```python
from build123d import *

# Parameters (mm, degrees)
SKETCH1_R           = 0.95
BOSS_EXTRUDE1_DEPTH = 3
SKETCH2_R           = 4
SKETCH2_R_2         = 0.95
BOSS_EXTRUDE2_DEPTH = 58


with BuildPart() as part:
    # Sketch1 → Boss-Extrude1 (new body)
    with BuildSketch(Plane(origin=(0, 0, 0), x_dir=(1, 0, 0), z_dir=(0, 1, 0))):
        with BuildLine():
            Line((-4.153311931, -5), (4.153311931, -5))
            ThreePointArc((4.153311931, -5), (6.5, 0), (4.153311931, 5))
            Line((4.153311931, 5), (-4.153311931, 5))
            ThreePointArc((-4.153311931, 5), (-6.5, 0), (-4.153311931, -5))
        make_face()
        with Locations(Location((0, 0, 0), (0, 0, 270))):
            Circle(SKETCH1_R, mode=Mode.SUBTRACT)
    extrude(amount=BOSS_EXTRUDE1_DEPTH)

    # Sketch2 → Boss-Extrude2 (add)
    with BuildSketch(Plane(origin=(0, 3, 0), x_dir=(1, 0, 0), z_dir=(0, 1, 0))):
        with Locations(Location((0, 0, 0), (0, 0, 90))):
            Circle(SKETCH2_R)
        with Locations(Location((0, 0, 0), (0, 0, 270))):
            Circle(SKETCH2_R_2, mode=Mode.SUBTRACT)
    extrude(amount=BOSS_EXTRUDE2_DEPTH)


solid = part.part
```
Check sheet for the modelled part. Datum: model origin and axes. Units: mm. A direction names the side the tool comes from. Coordinates: 2 decimals unless noted, no trailing zeros. Order: outer loops, then holes, each group sorted by start corner. A loop starts at its lowest first (then second) coordinate and runs counter-clockwise, first axis right, second up. Notation, with made-up numbers: M -35,60.25 L -12,60.25 A20 cw -12,96.25 Z; hole C 0.5,1.5 d2. An arc over 180 degrees is marked long. One line per question, with ' | ' between items. Start each with the question number.
Item 1: Sectioned sample at A-A on z = 0. Record the cut outline in (x, y).
Item 2: Sectioned sample at D-D on z = -3.25. Record the cut outline in (x, y), and give its area (3 significant figures).
Item 3: Gauge pin test, flat ends, axial feed: P1, Ø2, axis at x = -2, y = 15, coming from the +Z side; P2, Ø1.5, axis at y = 21.5, z = 0, coming from the -X side; P3, Ø1.5, axis at y = 14, z = -2, coming from the +X side. Record the tip position at first contact, or that the pin passes through.
Item 4: Mould release check, pull along Z, two halves, no side actions. Record for faces 3 (the cylindrical face through (-0.36, 30.07, 0.88)), 4 (the flat face through (0, 1, 5)), 5 (the flat face through (1, 61, -1)): pulls with the +Z half, pulls with the -Z half, needs draft (parallel to the pull), parting line crosses it, or undercut.
Item 5: Sectioned sample at B-B on x = 0. Record the cut outline in (y, z).
Item 6: Sectioned sample at C-C on y = 34. Record the cut outline in (x, z).
Item 7: Access from +Z, -Z, +X, -X, +Y, -Y to the whole of each face (thin tool, end or side, straight path). Record for faces 1 (the flat face through (-4.4, 3, -0.1)), 2 (the cylindrical face through (6.5, 1.5, 0.1)).
Item 8: Material ranges on line 1 (X direction, y = 14, z = 0); line 2 (Y direction, x = -3.5, z = 3); line 3 (Z direction, x = -0.5, y = 43), recorded low to high.
Answer below:
1) outline: M -6.5,0 L -0.95,0 L -0.95,61 L -4,61 L -4,3 L -6.5,3 Z; M 0.95,0 L 6.5,0 L 6.5,3 L 4,3 L 4,61 L 0.95,61 Z
2) outline: M -5.63,0 L 5.63,0 L 5.63,3 L 2.33,3 L 2.33,61 L -2.33,61 L -2.33,3 L -5.63,3 Z | area: 304 mm^2
3) P1: stops at z = 3.87 | P2: stops at x = -4 | P3: stops at x = 3.8
4) face 3: undercut | face 4: pulls with the +Z half | face 5: needs draft
5) outline: M 0,-5 L 3,-5 L 3,-4 L 61,-4 L 61,-0.95 L 0,-0.95 Z; M 0,0.95 L 61,0.95 L 61,4 L 3,4 L 3,5 L 0,5 Z
6) outline: C 0,0 d8; hole C 0,0 d1.9
7) face 1: +Y | face 2: +X, +Y, -Y
8) line 1: x = -4 to -0.95, 0.95 to 4 | line 2: y = 0 to 3 | line 3: z = -3.97 to -0.81, 0.81 to 3.97
